Autodesk Inventor part; units mm, degrees
ref_plane "YZ Plane" through (0, 0, 0) normal (1, 0, 0) x (0, 1, 0)
ref_plane "XZ Plane" through (0, 0, 0) normal (0, 1, 0) x (-1, 0, 0)
ref_plane "XY Plane" through (0, 0, 0) normal (0, 0, 1) x (1, 0, 0)
sketch "Sketch1" plane through (0, 0, 0) normal (0, 0, 1) x (1, 0, 0)
  line L0 (97.5839, -20.2585) -> (97.5839, -84.5585) construction
  line L1 (97.5839, -52.4085) -> (19.6066, -52.4085)
  line L2 (622.5839, -227.4085) -> (-427.4161, -227.4085)
  line L3 (-427.4161, -227.4085) -> (-427.4161, 122.5915)
  line L4 (-427.4161, 122.5915) -> (622.5839, 122.5915)
  line L5 (622.5839, 122.5915) -> (622.5839, -227.4085)
  line L6 (622.5839, -227.4085) -> (-427.4161, 122.5915) construction
  line L7 (-427.4161, -227.4085) -> (622.5839, 122.5915) construction
  line L8 (122.536, -54.5185) -> (122.536, 53.9215)
  line L9 (122.536, 53.9215) -> (107.7839, 53.9215)
  line L10 (107.7839, 53.9215) -> (107.7839, -54.5185)
  line L11 (107.7839, -54.5185) -> (122.536, -54.5185)
  line L12 (122.5839, -162.9585) -> (122.5839, -54.5185)
  line L13 (122.5839, -54.5185) -> (107.7839, -54.5185)
  line L14 (107.7839, -54.5185) -> (107.7839, -162.9585)
  line L15 (107.7839, -162.9585) -> (122.5839, -162.9585)
  line L16 (12.536, -54.5185) -> (12.536, 53.9215)
  line L17 (12.536, 53.9215) -> (-2.2161, 53.9215)
  line L18 (-2.2161, 53.9215) -> (-2.2161, -54.5185)
  line L19 (-2.2161, -54.5185) -> (12.536, -54.5185)
  line L20 (12.5839, -162.9585) -> (12.5839, -54.5185)
  line L21 (12.5839, -54.5185) -> (-2.2161, -54.5185)
  line L22 (-2.2161, -54.5185) -> (-2.2161, -162.9585)
  line L23 (-2.2161, -162.9585) -> (12.5839, -162.9585)
  line L24 (-97.4161, -162.9585) -> (-97.4161, -54.5185)
  line L25 (-97.4161, -54.5185) -> (-112.2161, -54.5185)
  line L26 (-112.2161, -54.5185) -> (-112.2161, -162.9585)
  line L27 (-112.2161, -162.9585) -> (-97.4161, -162.9585)
  line L28 (-97.464, -54.5185) -> (-97.464, 53.9215)
  line L29 (-97.464, 53.9215) -> (-112.2161, 53.9215)
  line L30 (-112.2161, 53.9215) -> (-112.2161, -54.5185)
  line L31 (-112.2161, -54.5185) -> (-97.464, -54.5185)
  line L32 (-317.464, -54.5185) -> (-317.464, 53.9215)
  line L33 (-317.464, 53.9215) -> (-332.2161, 53.9215)
  line L34 (-332.2161, 53.9215) -> (-332.2161, -54.5185)
  line L35 (-332.2161, -54.5185) -> (-317.464, -54.5185)
  line L36 (-317.4161, -162.9585) -> (-317.4161, -54.5185)
  line L37 (-317.4161, -54.5185) -> (-332.2161, -54.5185)
  line L38 (-332.2161, -54.5185) -> (-332.2161, -162.9585)
  line L39 (-332.2161, -162.9585) -> (-317.4161, -162.9585)
  line L40 (-207.4161, -162.9585) -> (-207.4161, -54.5185)
  line L41 (-207.4161, -54.5185) -> (-222.2161, -54.5185)
  line L42 (-222.2161, -54.5185) -> (-222.2161, -162.9585)
  line L43 (-222.2161, -162.9585) -> (-207.4161, -162.9585)
  line L44 (-207.464, -54.5185) -> (-207.464, 53.9215)
  line L45 (-207.464, 53.9215) -> (-222.2161, 53.9215)
  line L46 (-222.2161, 53.9215) -> (-222.2161, -54.5185)
  line L47 (-222.2161, -54.5185) -> (-207.464, -54.5185)
  line L48 (562.536, -54.5185) -> (562.536, 53.9215)
  line L49 (562.536, 53.9215) -> (547.7839, 53.9215)
  line L50 (547.7839, 53.9215) -> (547.7839, -54.5185)
  line L51 (547.7839, -54.5185) -> (562.536, -54.5185)
  line L52 (562.5839, -162.9585) -> (562.5839, -54.5185)
  line L53 (562.5839, -54.5185) -> (547.7839, -54.5185)
  line L54 (547.7839, -54.5185) -> (547.7839, -162.9585)
  line L55 (547.7839, -162.9585) -> (562.5839, -162.9585)
  line L56 (452.5839, -162.9585) -> (452.5839, -54.5185)
  line L57 (452.5839, -54.5185) -> (437.7839, -54.5185)
  line L58 (437.7839, -54.5185) -> (437.7839, -162.9585)
  line L59 (437.7839, -162.9585) -> (452.5839, -162.9585)
  line L60 (452.536, -54.5185) -> (452.536, 53.9215)
  line L61 (452.536, 53.9215) -> (437.7839, 53.9215)
  line L62 (437.7839, 53.9215) -> (437.7839, -54.5185)
  line L63 (437.7839, -54.5185) -> (452.536, -54.5185)
  line L64 (342.536, -54.5185) -> (342.536, 53.9215)
  line L65 (342.536, 53.9215) -> (327.7839, 53.9215)
  line L66 (327.7839, 53.9215) -> (327.7839, -54.5185)
  line L67 (327.7839, -54.5185) -> (342.536, -54.5185)
  line L68 (342.5839, -162.9585) -> (342.5839, -54.5185)
  line L69 (342.5839, -54.5185) -> (327.7839, -54.5185)
  line L70 (327.7839, -54.5185) -> (327.7839, -162.9585)
  line L71 (327.7839, -162.9585) -> (342.5839, -162.9585)
  line L72 (232.536, -54.5185) -> (232.536, 53.9215)
  line L73 (232.536, 53.9215) -> (217.7839, 53.9215)
  line L74 (217.7839, 53.9215) -> (217.7839, -54.5185)
  line L75 (217.7839, -54.5185) -> (232.536, -54.5185)
  line L76 (232.5839, -162.9585) -> (232.5839, -54.5185)
  line L77 (232.5839, -54.5185) -> (217.7839, -54.5185)
  line L78 (217.7839, -54.5185) -> (217.7839, -162.9585)
  line L79 (217.7839, -162.9585) -> (232.5839, -162.9585)
  line L80 (144.8839, -131.8585) -> (144.8839, -227.4085)
  line L81 (140.5839, -227.4085) -> (140.5839, -131.8585)
  arc A0 (144.8839, -131.8585) -> (97.5839, -84.5585) centre (97.5839, -131.8585) ccw
  arc A1 (140.5839, -131.8585) -> (97.5839, -88.8585) centre (97.5839, -131.8585) ccw
  line L82 (-34.764, -227.4085) -> (-34.764, -63.2585)
  line L83 (-30.464, -63.2585) -> (-30.464, -227.4085)
  arc A2 (12.536, -20.2585) -> (-30.464, -63.2585) centre (12.536, -63.2585) ccw
  arc A3 (12.536, -15.9585) -> (-34.764, -63.2585) centre (12.536, -63.2585) ccw
  circle A4 centre (-417.4161, 112.5915) radius 3
  line L84 (622.5839, 122.5915) -> (-427.4161, 122.5915)
  line L85 (622.5839, -227.4085) -> (622.5839, 122.5915)
  line L86 (-427.4161, -227.4085) -> (622.5839, -227.4085)
  line L87 (-427.4161, 122.5915) -> (-427.4161, -227.4085)
  circle A5 centre (-417.4161, -217.4085) radius 3
  line L88 (622.5839, 122.5915) -> (-427.4161, 122.5915)
  line L89 (622.5839, -227.4085) -> (622.5839, 122.5915)
  line L90 (-427.4161, -227.4085) -> (622.5839, -227.4085)
  line L91 (-427.4161, 122.5915) -> (-427.4161, -227.4085)
  line L92 (622.5839, 122.5915) -> (-427.4161, 122.5915)
  line L93 (622.5839, -227.4085) -> (622.5839, 122.5915)
  line L94 (-427.4161, -227.4085) -> (622.5839, -227.4085)
  line L95 (-427.4161, 122.5915) -> (-427.4161, -227.4085)
  circle A6 centre (612.5839, 112.5915) radius 3
  circle A7 centre (612.5839, -217.4085) radius 3
  circle A8 centre (-159.9161, -217.4085) radius 3
  circle A9 centre (97.5839, -217.4085) radius 3
  circle A10 centre (355.0839, -217.4085) radius 3
  circle A11 centre (-159.9161, 112.5915) radius 3
  circle A12 centre (97.5839, 112.5915) radius 3
  circle A13 centre (355.0839, 112.5915) radius 3
  circle A14 centre (97.5839, 112.5915) radius 3
  circle A15 centre (612.5839, -217.4085) radius 3
  circle A16 centre (355.0839, -217.4085) radius 3
  circle A17 centre (97.5839, -217.4085) radius 3
  circle A18 centre (-159.9161, -217.4085) radius 3
  circle A19 centre (-417.4161, -217.4085) radius 3
  circle A20 centre (355.0839, 112.5915) radius 3
  circle A21 centre (-417.4161, 112.5915) radius 3
  circle A22 centre (612.5839, 112.5915) radius 3
  circle A23 centre (-159.9161, 112.5915) radius 3
  circle A24 centre (97.5839, 112.5915) radius 3
  circle A25 centre (612.5839, -217.4085) radius 3
  circle A26 centre (355.0839, -217.4085) radius 3
  circle A27 centre (97.5839, -217.4085) radius 3
  circle A28 centre (-159.9161, -217.4085) radius 3
  circle A29 centre (-417.4161, -217.4085) radius 3
  circle A30 centre (355.0839, 112.5915) radius 3
  circle A31 centre (-417.4161, 112.5915) radius 3
  circle A32 centre (612.5839, 112.5915) radius 3
  circle A33 centre (-159.9161, 112.5915) radius 3
  circle A34 centre (97.5839, 112.5915) radius 3
  circle A35 centre (612.5839, -217.4085) radius 3
  circle A36 centre (355.0839, -217.4085) radius 3
  circle A37 centre (97.5839, -217.4085) radius 3
  circle A38 centre (-159.9161, -217.4085) radius 3
  circle A39 centre (-417.4161, -217.4085) radius 3
  circle A40 centre (355.0839, 112.5915) radius 3
  circle A41 centre (-417.4161, 112.5915) radius 3
  circle A42 centre (612.5839, 112.5915) radius 3
  circle A43 centre (-159.9161, 112.5915) radius 3
  point P0 (0, 0)
  point P1 (-2.2161, -18.3178)
  point P2 (-2.2161, -22.8682)
  point P3 (122.5839, -96.8728)
  point P4 (122.5839, -91.7052)
  dimension "d0" = 1050
  dimension "d1" = 350
extrude "Extrusion2" add sketch "Sketch1" along normal blind 8.5 contours L2 L80 A0 L12 L13 L8 L9 L10 L14 L15 A1 L81 L83 A2 L18 L22 L23 L20 L21 L16 L17 A3 L82 L3 L4 L5
sketch "Sketch2" plane through (144.8839, -227.4085, 0) normal (-1, 0, 0) x (0, 0, 1)
  line L0 (0, 95.55) -> (8.5, 95.55)
  line L1 (0, 95.55) -> (0, 0)
  line L2 (0, 0) -> (8.5, 0)
  line L3 (8.5, 95.55) -> (8.5, 0)
  line L4 (4.2, 0) -> (4.2, 95.55)
  point P0 (0, 227.4085)
  dimension "d6" = 4.3
  dimension "d7" = 4.3
extrude "Extrusion3" add sketch "Sketch2" along normal blind 4.3 contours L0 L4 L2 L1
sketch "Sketch3" plane through (-34.764, -227.4085, 0) normal (1, 0, 0) x (0, 0, -1)
  line L0 (0, 0) -> (0, 164.15)
  line L1 (0, 164.15) -> (-8.5, 164.15)
  line L2 (-8.5, 0) -> (-8.5, 164.15)
  line L3 (0, 0) -> (-8.5, 0)
  line L4 (0, 164.15) -> (-8.5, 164.15)
  line L5 (-4.2, 164.15) -> (-4.2, 0)
  point P0 (0, 227.4085)
  dimension "d10" = 4.3
  dimension "d11" = 4.3
extrude "Extrusion4" add sketch "Sketch3" along normal blind 4.3 contours L3 L5 L1 L0
properties part number "PrimaryCoilFerriteLayer" material "Iron, Cast"
The model under review builds one solid part; all positions refer to its coordinate system, in mm. A direction names the side the tool comes from. Give positions to 0.01 mm unless a question says otherwise; leave off trailing zeros. Write each question's results on one line, items separated by ' | '. Start each with the question number.
1. We need section A-A (y = -9). Count the separate pieces of the cut face and the enclosed holes in it, and give its area (3 significant figures).
2. Mouldability with a two-part tool opening along X and no side actions: class faces 3 (the flat face through (90, -50, 8.5)), 4 (the cylindrical face through (138.77, -108.6, 4.19)) as released by +X, released by -X, zero draft, split by the parting line, or undercut.
3. For faces 1 (the cylindrical face through (-26.014, -35.851, 4.19)), 2 (the flat face through (90, -55, 0)), list the 3-axis set-ups (+Z, -Z, +X, -X, +Y, -Y) from which the entire face can be reached by the end or side of a thin tool; tool diameter is ignored.
4. For probe 1 along Y at (x, z) = (-0.5, 7); probe 2 along Y at (x, z) = (352.5, 6.25), list the stretches that pass through material, from the lowest coordinate up. Write a range as [from, to].
Results found:
1) separate pieces: 10 | enclosed holes: 0 | area: 7,800 mm^2
2) face 3: zero draft | face 4: undercut
3) face 1: +Z, -Z | face 2: -Z, +X, -X, +Y, -Y
4) probe 1: y = [-227.41, -162.96], [53.92, 122.59] | probe 2: y = [-227.41, -218.93], [-215.88, 111.07], [114.12, 122.59]
